```python
from build123d import *

# Parameters (mm, degrees)
SKETCH_1_R          = 54
SKETCH_1_R_2        = 50.5
EXTRUDE_1_DEPTH     = 230
SKETCH_2_R          = 51.5
CUT_EXTRUDE_1_DEPTH = 5
SKETCH_3_R          = 7.5
CUT_EXTRUDE_2_DEPTH = 101


with BuildPart() as part:
    # Эскиз1 → Бобышка-Вытянуть1 (new body)
    with BuildSketch(Plane(origin=(0, 0, 0), x_dir=(1, 0, 0), z_dir=(0, 1, 0))):
        with Locations(Location((0, 0, 0), (0, 0, 270))):
            Circle(SKETCH_1_R)
        with Locations(Location((0, 0, 0), (0, 0, 270))):
            Circle(SKETCH_1_R_2, mode=Mode.SUBTRACT)
    extrude(amount=EXTRUDE_1_DEPTH)

    # Эскиз2 → Вырез-Вытянуть1 (cut)
    with BuildSketch(Plane(origin=(0, 230, 0), x_dir=(1, 0, 0), z_dir=(0, 1, 0))):
        with Locations(Location((0, 0, 0), (0, 0, 270))):
            Circle(SKETCH_2_R)
    extrude(amount=-CUT_EXTRUDE_1_DEPTH, mode=Mode.SUBTRACT)

    # Эскиз3 → Вырез-Вытянуть2 (cut)
    with BuildSketch(Plane.XY):
        with Locations(Location((0, 115, 0), (0, 0, 180))):
            Circle(SKETCH_3_R)
    extrude(amount=CUT_EXTRUDE_2_DEPTH, mode=Mode.SUBTRACT)


solid = part.part
```
Geometry check sheet. Reference: the model listing, model coordinates, mm. Round coordinates to 2 decimals unless told otherwise and drop trailing zeros. Order: outer loops, then holes, each group sorted by start corner. A loop starts at its lowest first (then second) coordinate and runs counter-clockwise, first axis right, second up. Notation, with made-up numbers: (13.5, 89) -> (21.5, 89) arc R11 cw to (21.5, 107) -> close; hole circle Ø5 at (-12.5, -20). An arc over 180 degrees is marked (long way). Return JSON: item names as keys, results as strings. Group by question number.
Q1. Section check B-B, the plane x = 0. Record the boundary of the cut face in (y, z).
Q2. Gauge pin test, flat ends, axial feed: pin 1 (1 mm diameter, centred on x = -34, y = 189, fed in from +Z); pin 2 (12 mm diameter, centred on y = 154, z = 30, fed in from +X); pin 3 (5 mm diameter, centred on x = 6, y = 123.5, fed in from -Z). Record the tip position at first contact, or that the pin passes through.
Q3. Section check A-A, the plane z = 0. Record the boundary of the cut face in (x, y).
Q4. Section check C-C, the plane x = -40.5. Record the boundary of the cut face in (y, z), plus the area to 3 significant figures.
Q5. Section check D-D, the plane y = 187. Record the boundary of the cut face in (x, z), plus the area to 3 significant figures.
Q6. Material ranges on probe 1 along X at (y, z) = (227, 0); probe 2 along Z at (x, y) = (-13, 59.5); probe 3 along X at (y, z) = (82.5, -2), recorded low to high. Write a range as from..to.
Q7. Release check for a two-part mould opening along Y. For faces 1 (the cylindrical face through (-45.69, 227.54, 23.76)), 2 (the cylindrical face through (-6.93, 117.87, 51.94)), 3 (the flat face through (-38, 225, 34)), 4 (the flat face through (-36, 0, 36)) record: released by +Y, released by -Y, zero draft, split by the parting line, or undercut.
Numbers:
{
 "1": {"outline": "(0, -54) -> (230, -54) -> (230, -51.5) -> (225, -51.5) -> (225, -50.5) -> (0, -50.5) -> close; (0, 50.5) -> (107.5, 50.5) -> (107.5, 54) -> (0, 54) -> close; (122.5, 50.5) -> (225, 50.5) -> (225, 51.5) -> (230, 51.5) -> (230, 54) -> (122.5, 54) -> close"},
 "2": {"pin 1": "z = 42.35", "pin 2": "x = 48.37", "pin 3": "z = -53.89"},
 "3": {"outline": "(-54, 0) -> (-50.5, 0) -> (-50.5, 225) -> (-51.5, 225) -> (-51.5, 230) -> (-54, 230) -> close; (50.5, 0) -> (54, 0) -> (54, 230) -> (51.5, 230) -> (51.5, 225) -> (50.5, 225) -> close"},
 "4": {"outline": "(0, -35.72) -> (230, -35.72) -> (230, -31.81) -> (225, -31.81) -> (225, -30.17) -> (0, -30.17) -> close; (0, 30.17) -> (225, 30.17) -> (225, 31.81) -> (230, 31.81) -> (230, 35.72) -> (0, 35.72) -> close", "area": "2,540 mm^2"},
 "5": {"outline": "circle Ø108 at (0, 0); hole circle Ø101 at (0, 0)", "area": "1,150 mm^2"},
 "6": {"probe 1": "-54..-51.5, 51.5..54", "probe 2": "-52.41..-48.8, 48.8..52.41", "probe 3": "-53.96..-50.46, 50.46..53.96"},
 "7": {"face 1": "zero draft", "face 2": "undercut", "face 3": "released by +Y", "face 4": "released by -Y"}
}
